Study the drawing (mm; zero at the part's minimum x, y, z) and answer. A direction names the side the tool comes from. Coordinates: 2 decimals unless noted, no trailing zeros. Write each loop counter-clockwise with the first axis right and the second up, starting at its lowest first coordinate (ties: lowest second). Pieces come first, ordered by that corner, then holes. Notation, with made-up numbers: (74, -6) -> (101, -6) arc R20 cw to (101, 26) -> close; hole circle Ø8 at (82.5, 75.25). An arc over 180 degrees is marked (long way). Write each question's results on one line, items separated by ' | '. Start each with the question number.
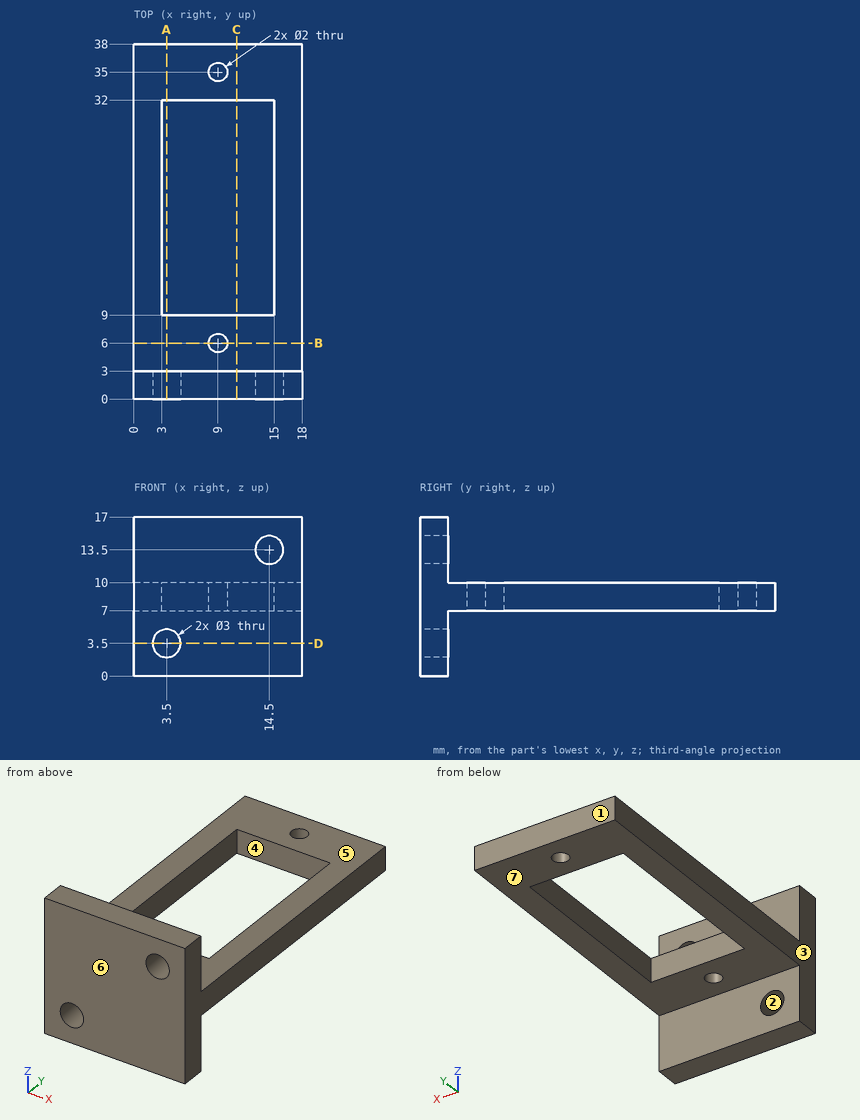
1. Determine the mould class of the marked faces 1, 2 and 3 for opening direction X: pulls with the +X half, pulls with the -X half, needs draft (parallel to the pull), parting line crosses it, or undercut.
2. For the marked faces 4, 5, 6 and 7, determine the directions among +Z, -Z, +X, -X, +Y, -Y from which every point of the face is accessible in a straight line to the end or side of a thin tool.
3. Given pin 1 Ø10 at (x, y) = (2.5, 11) entering from +Z; pin 2 Ø8 at (x, z) = (12.5, 11.5) entering from -Y; pin 3 Ø3.5 at (x, z) = (6.5, 4) entering from +Y; pin 4 Ø2.5 at (x, y) = (9, 35) entering from -Z, each flat-ended and moving along its own axis, determine where each tip first touches the part or whether it passes through.
4. Find the intervals of material crossed by L1, parallel to Y at x = 9, z = 8.45; L2, parallel to Z at x = 14.5, y = 0.7; L3, parallel to Y at x = 9.25, z = 6.5, in increasing order.
5. Find section A-A on x = 3.5. Give the vertices of the cut face in (y, z).
6. Find section C-C on x = 11. Give the vertices of the cut face in (y, z).
7. Find section D-D on z = 3.5. Give the vertices of the cut face in (x, y).
8. Find section B-B on y = 6. Give the vertices of the cut face in (x, z).
Ans:
1) face 1: needs draft | face 2: undercut | face 3: pulls with the -X half
2) face 4: +Z, -Z | face 5: +Z, +X, -X, +Y | face 6: +Z, -Z, +X, -X, -Y | face 7: -Z, +X, -X, +Y
3) pin 1: stops at z = 10 | pin 2: stops at y = 0 | pin 3: stops at y = 3 | pin 4: stops at z = 7
4) L1: y = 0 to 5, 7 to 9, 32 to 34, 36 to 38 | L2: z = 0 to 12, 15 to 17 | L3: y = 0 to 3
5) outline: (0, 0) -> (3, 0) -> (3, 2) -> (0, 2) -> close; (0, 5) -> (3, 5) -> (3, 7) -> (9, 7) -> (9, 10) -> (3, 10) -> (3, 17) -> (0, 17) -> close; (32, 7) -> (38, 7) -> (38, 10) -> (32, 10) -> close
6) outline: (0, 0) -> (3, 0) -> (3, 7) -> (9, 7) -> (9, 10) -> (3, 10) -> (3, 17) -> (0, 17) -> close; (32, 7) -> (38, 7) -> (38, 10) -> (32, 10) -> close
7) outline: (0, 0) -> (2, 0) -> (2, 3) -> (0, 3) -> close; (5, 0) -> (18, 0) -> (18, 3) -> (5, 3) -> close
8) outline: (0, 7) -> (8, 7) -> (8, 10) -> (0, 10) -> close; (10, 7) -> (18, 7) -> (18, 10) -> (10, 10) -> close
